For this review, take the finished solid that the model builds, in its own axes (mm). A direction names the side the tool comes from. Round coordinates to 2 decimals unless told otherwise and drop trailing zeros. Loops run counter-clockwise (first coordinate to the right, second up) from the corner with the lowest first, then second, coordinate; pieces in that order, holes last.
1. Clearance check with flat-ended pins moving along their axes: pin 1 Ø6.5 at (y, z) = (13.5, 39) entering from +X; pin 2 Ø17.5 at (y, z) = (14, 37) entering from -X; pin 3 Ø17.5 at (y, z) = (22.5, -82) entering from -X. State where each tip first meets the part, or that it passes through.
2. Draft analysis for pull direction Z (two halves, no side actions). For faces 4 (the cylindrical face through (99.863, 20.995, 39.854)), 5 (the flat face through (-3, 99, -139.184)), 6 (the flat face through (-3, 0, 96)), 7 (the cylindrical face through (96.849, 18.995, -70.102)), state which applies: released by +Z, released by -Z, zero draft, split by the parting line, or undercut.
3. To check wall thickness, follow line 1 along X through (y, z) = (19, 10.5); line 2 along Z through (x, y) = (-15, 11); line 3 along Z through (x, y) = (48, 37). State the ranges of each line that lie inside material, in increasing order.
4. Consider section C-C on x = 15.5. State the section outline as (y, z) points, then the cut area to 3 significant figures.
5. Consider section B-B on z = 0. State the section outline as (x, y) points.
6. Tool access review of faces 1 (the cylindrical face through (102.602, 18.995, 39.898)), 2 (the cylindrical face through (-103, 33, -70)), 3 (the cylindrical face through (-86, 31, 40)): name each direction out of +Z, -Z, +X, -X, +Y, -Y from which nothing blocks a thin tool from reaching the whole face with its end or side.
7. Consider section A-A on x = -68.5. State the section outline as (y, z) points.
from build123d import *

# Parameters (mm, degrees)
F1_DEPTH = 200


with BuildPart() as f1:
    # F0 (on Front) → F1 (new body)
    with BuildSketch(Plane.XZ):
        Polygon((-107.723215, 71.316256), (-107.723215, 40.316256), (104.376785, 40.316256), (104.376785, 59.316256), (100.876785, 59.316256), (100.876785, 61.316256), (98.876785, 61.316256), (98.876785, 59.316256), (94.876785, 59.316256), (94.876785, 67.316256), (93.876785, 67.316256), (93.876785, 71.316256), (77.576785, 71.316256), (77.576785, 89.816256), (21.276785, 89.816256), (21.276785, 71.316256), (-23.923215, 71.316256), (-23.923215, 89.816256), (-80.223215, 89.816256), (-80.223215, 71.316256), (-90.723215, 71.316256), (-90.723215, 74.916256), (-92.723215, 74.916256), (-92.723215, 71.316256), (-101.723215, 71.316256), (-101.723215, 73.316256), (-103.723215, 73.316256), (-103.723215, 71.316256), align=None)
        Polygon((-107.723215, 109.816256), (-107.723215, 71.316256), (-103.723215, 71.316256), (-103.723215, 73.316256), (-101.723215, 73.316256), (-101.723215, 71.316256), (-92.723215, 71.316256), (-92.723215, 74.916256), (-90.723215, 74.916256), (-90.723215, 71.316256), (-80.223215, 71.316256), (-80.223215, 89.816256), (-23.923215, 89.816256), (-23.923215, 71.316256), (21.276785, 71.316256), (21.276785, 89.816256), (77.576785, 89.816256), (77.576785, 71.316256), (93.876785, 71.316256), (93.876785, 67.316256), (94.876785, 67.316256), (94.876785, 59.316256), (98.876785, 59.316256), (98.876785, 61.316256), (100.876785, 61.316256), (100.876785, 59.316256), (104.376785, 59.316256), (104.376785, 109.816256), align=None)
        Polygon((-107.723215, 40.316256), (-107.723215, 9.316256), (-103.723215, 9.316256), (-103.723215, 7.316256), (-101.723215, 7.316256), (-101.723215, 9.316256), (-92.723215, 9.316256), (-92.723215, 5.716256), (-90.723215, 5.716256), (-90.723215, 9.316256), (-80.223215, 9.316256), (-80.223215, -9.183744), (-23.923215, -9.183744), (-23.923215, 9.316256), (21.276785, 9.316256), (21.276785, -9.183744), (77.576785, -9.183744), (77.576785, 9.316256), (93.876785, 9.316256), (93.876785, 13.316256), (94.876785, 13.316256), (94.876785, 21.316256), (98.876785, 21.316256), (98.876785, 19.316256), (100.876785, 19.316256), (100.876785, 21.316256), (104.376785, 21.316256), (104.376785, 40.316256), align=None)
        Polygon((-107.723215, 9.316256), (-107.723215, -38.683744), (-103.723215, -38.683744), (-103.723215, -36.683744), (-101.723215, -36.683744), (-101.723215, -38.683744), (-92.723215, -38.683744), (-92.723215, -35.083744), (-90.723215, -35.083744), (-90.723215, -38.683744), (-80.223215, -38.683744), (-80.223215, -20.183744), (-23.923215, -20.183744), (-23.923215, -38.683744), (21.276785, -38.683744), (21.276785, -20.183744), (77.576785, -20.183744), (77.576785, -38.683744), (93.876785, -38.683744), (93.876785, -42.683744), (94.876785, -42.683744), (94.876785, -50.683744), (98.876785, -50.683744), (98.876785, -48.683744), (100.876785, -48.683744), (100.876785, -50.683744), (104.376785, -50.683744), (104.376785, 21.316256), (100.876785, 21.316256), (100.876785, 19.316256), (98.876785, 19.316256), (98.876785, 21.316256), (94.876785, 21.316256), (94.876785, 13.316256), (93.876785, 13.316256), (93.876785, 9.316256), (77.576785, 9.316256), (77.576785, -9.183744), (21.276785, -9.183744), (21.276785, 9.316256), (-23.923215, 9.316256), (-23.923215, -9.183744), (-80.223215, -9.183744), (-80.223215, 9.316256), (-90.723215, 9.316256), (-90.723215, 5.716256), (-92.723215, 5.716256), (-92.723215, 9.316256), (-101.723215, 9.316256), (-101.723215, 7.316256), (-103.723215, 7.316256), (-103.723215, 9.316256), align=None)
        Polygon((-103.723215, -38.683744), (-107.723215, -38.683744), (-107.723215, -69.683744), (104.376785, -69.683744), (104.376785, -50.683744), (100.876785, -50.683744), (100.876785, -48.683744), (98.876785, -48.683744), (98.876785, -50.683744), (94.876785, -50.683744), (94.876785, -42.683744), (93.876785, -42.683744), (93.876785, -38.683744), (77.576785, -38.683744), (77.576785, -20.183744), (21.276785, -20.183744), (21.276785, -38.683744), (-23.923215, -38.683744), (-23.923215, -20.183744), (-80.223215, -20.183744), (-80.223215, -38.683744), (-90.723215, -38.683744), (-90.723215, -35.083744), (-92.723215, -35.083744), (-92.723215, -38.683744), (-101.723215, -38.683744), (-101.723215, -36.683744), (-103.723215, -36.683744), align=None)
        Polygon((104.376785, -69.683744), (-107.723215, -69.683744), (-107.723215, -100.683744), (-103.723215, -100.683744), (-103.723215, -102.683744), (-101.723215, -102.683744), (-101.723215, -100.683744), (-92.723215, -100.683744), (-92.723215, -104.283744), (-90.723215, -104.283744), (-90.723215, -100.683744), (-80.223215, -100.683744), (-80.223215, -119.183744), (-23.923215, -119.183744), (-23.923215, -100.683744), (21.276785, -100.683744), (21.276785, -119.183744), (77.576785, -119.183744), (77.576785, -100.683744), (93.876785, -100.683744), (93.876785, -96.683744), (94.876785, -96.683744), (94.876785, -88.683744), (98.876785, -88.683744), (98.876785, -90.683744), (100.876785, -90.683744), (100.876785, -88.683744), (104.376785, -88.683744), align=None)
        Polygon((-103.723215, -100.683744), (-107.723215, -100.683744), (-107.723215, -139.183744), (104.376785, -139.183744), (104.376785, -88.683744), (100.876785, -88.683744), (100.876785, -90.683744), (98.876785, -90.683744), (98.876785, -88.683744), (94.876785, -88.683744), (94.876785, -96.683744), (93.876785, -96.683744), (93.876785, -100.683744), (77.576785, -100.683744), (77.576785, -119.183744), (21.276785, -119.183744), (21.276785, -100.683744), (-23.923215, -100.683744), (-23.923215, -119.183744), (-80.223215, -119.183744), (-80.223215, -100.683744), (-90.723215, -100.683744), (-90.723215, -104.283744), (-92.723215, -104.283744), (-92.723215, -100.683744), (-101.723215, -100.683744), (-101.723215, -102.683744), (-103.723215, -102.683744), align=None)
    extrude(amount=-F1_DEPTH)

    # F0 (on Front) → F2 (revolve, cut)
    with BuildSketch(Plane.XZ):
        Polygon((-107.723215, 71.316256), (-107.723215, 40.316256), (104.376785, 40.316256), (104.376785, 59.316256), (100.876785, 59.316256), (100.876785, 61.316256), (98.876785, 61.316256), (98.876785, 59.316256), (94.876785, 59.316256), (94.876785, 67.316256), (93.876785, 67.316256), (93.876785, 71.316256), (77.576785, 71.316256), (77.576785, 89.816256), (21.276785, 89.816256), (21.276785, 71.316256), (-23.923215, 71.316256), (-23.923215, 89.816256), (-80.223215, 89.816256), (-80.223215, 71.316256), (-90.723215, 71.316256), (-90.723215, 74.916256), (-92.723215, 74.916256), (-92.723215, 71.316256), (-101.723215, 71.316256), (-101.723215, 73.316256), (-103.723215, 73.316256), (-103.723215, 71.316256), align=None)
    revolve(axis=Axis((-1.673215, 0, 40.316256), (1, 0, 0)), mode=Mode.SUBTRACT)

    # F0 (on Front) → F3 (revolve, cut)
    with BuildSketch(Plane.XZ):
        Polygon((-103.723215, -38.683744), (-107.723215, -38.683744), (-107.723215, -69.683744), (104.376785, -69.683744), (104.376785, -50.683744), (100.876785, -50.683744), (100.876785, -48.683744), (98.876785, -48.683744), (98.876785, -50.683744), (94.876785, -50.683744), (94.876785, -42.683744), (93.876785, -42.683744), (93.876785, -38.683744), (77.576785, -38.683744), (77.576785, -20.183744), (21.276785, -20.183744), (21.276785, -38.683744), (-23.923215, -38.683744), (-23.923215, -20.183744), (-80.223215, -20.183744), (-80.223215, -38.683744), (-90.723215, -38.683744), (-90.723215, -35.083744), (-92.723215, -35.083744), (-92.723215, -38.683744), (-101.723215, -38.683744), (-101.723215, -36.683744), (-103.723215, -36.683744), align=None)
    revolve(axis=Axis((-1.673215, 0, -69.683744), (1, 0, 0)), mode=Mode.SUBTRACT)


solid = f1.part
Resolved:
1. pin 1: passes through
1. pin 2: stops at x = 94.88
1. pin 3: stops at x = -107.72
2. face 4: undercut
2. face 5: released by -Z
2. face 6: zero draft
2. face 7: undercut
3. line 1: x = -107.72 to -80.22, -23.92 to 21.28, 77.58 to 104.38
3. line 2: z = -139.18 to -98.67, -40.7 to 11.33, 69.3 to 109.82
3. line 3: z = -139.18 to -102.57, -36.8 to 7.43, 73.2 to 109.82
4. outline: (0, -139.18) - (200, -139.18) - (200, 109.82) - (0, 109.82) - (0, 71.32) arc R31 cw to (0, 9.32) - (0, -38.68) arc R31 cw to (0, -100.68) - close
4. area: 46,800 mm2
5. outline: (-107.72, 0) - (-80.22, 0) - (-80.22, 28.72) - (-23.92, 28.72) - (-23.92, 0) - (21.28, 0) - (21.28, 28.72) - (77.58, 28.72) - (77.58, 0) - (104.38, 0) - (104.38, 200) - (-107.72, 200) - close
6. face 1: +X, -X, -Y
6. face 2: -Y
6. face 3: -X, -Y
7. outline: (0, -139.18) - (200, -139.18) - (200, 109.82) - (0, 109.82) - (0, 89.82) arc R49.5 cw to (0, -9.18) - (0, -20.18) arc R49.5 cw to (0, -119.18) - close
